Autodesk Inventor part; units mm, degrees
ref_plane "XZ Plane" through (0, 0, 0) normal (0, 1, 0) x (-1, 0, 0)
sketch "Szkic1" plane through (0, 0, 0) normal (0, 1, 0) x (-1, 0, 0)
  circle A0 centre (0, 0) radius 1.75
  dimension "d0" = 3.5
extrude "Wyciągnięcie proste1" add sketch "Szkic1" along normal blind 8
sketch "Szkic2" plane through (0, 8, 0) normal (0, 1, 0) x (1, 0, 0)
  circle A0 centre (0, 0) radius 3
  dimension "d3" = 6
extrude "Wyciągnięcie proste2" add sketch "Szkic2" along normal blind 70
sketch "Szkic3" plane through (0, 78, 0) normal (0, 1, 0) x (1, 0, 0)
  circle A0 centre (0, 0) radius 1.75
  circle A1 centre (0, 0) radius 1.75
  dimension "d6" = 3.5
extrude "Wyciągnięcie proste3" add sketch "Szkic3" along normal blind 8
properties part number "rod_longer"
Could you check a few things on this model? Use its own coordinates, in mm. A direction names the side the tool comes from. Give positions to 0.01 mm unless a question says otherwise; leave off trailing zeros. Order: outer loops, then holes, each group sorted by start corner. A loop starts at its lowest first (then second) coordinate and runs counter-clockwise, first axis right, second up. Notation, with made-up numbers: (88.5, -24.5) - (147.5, -24.5) arc R15 cw to (147.5, -5.5) - close; hole circle Ø5 at (39, -20). An arc over 180 degrees is marked (long way). One line per item, written item: value. Start each with the question number.
1. If I drill on probe 1 along X at (y, z) = (60, -0.1); probe 2 along Y at (x, z) = (0.6, 1.75); probe 3 along Z at (x, y) = (2.4, 70), over which ranges is the centre line in solid material (lowest first)?
2. Imagine slicing it at B-B on x = 0. List the corners of the cut face in (y, z) for me.
3. Imagine slicing it at C-C on y = 16.5. List the corners of the cut face in (x, z) for me.
4. For faces 1 (the face through (-1.617, 3.944, 0.67)), 2 (the face through (-3, 43, 0)), 3 (the face through (1.617, 81.944, -0.67)), which set-ups out of +Z, -Z, +X, -X, +Y, -Y let a thin tool reach every point of the face, with its end or its side?
5. For P1, Ø1.5, axis at x = -2.5, y = 28, coming from the +Z side; P2, Ø1.8, axis at x = 0.5, z = 0, coming from the -Y side, each with a flat end and sliding along its axis, tell me the tip position at first contact or that it passes through.
6. Imagine slicing it at A-A on z = 0. List the corners of the cut face in (x, y) for me.
Values:
1. probe 1: -3 to 3
1. probe 2: 8 to 78
1. probe 3: -1.8 to 1.8
2. outline: (0, -1.75) - (8, -1.75) - (8, -3) - (78, -3) - (78, -1.75) - (86, -1.75) - (86, 1.75) - (78, 1.75) - (78, 3) - (8, 3) - (8, 1.75) - (0, 1.75) - close
3. outline: circle Ø6 at (0, 0)
4. face 1: -Y
4. face 2: +Y, -Y
4. face 3: +Y
5. P1: z = 2.44
5. P2: y = 0
6. outline: (-3, 8) - (-1.75, 8) - (-1.75, 0) - (1.75, 0) - (1.75, 8) - (3, 8) - (3, 78) - (1.75, 78) - (1.75, 86) - (-1.75, 86) - (-1.75, 78) - (-3, 78) - close
